The model under review builds one solid part; all positions refer to its coordinate system, in mm. A direction names the side the tool comes from. Round coordinates to 2 decimals unless told otherwise and drop trailing zeros. Order: outer loops, then holes, each group sorted by start corner. A loop starts at its lowest first (then second) coordinate and runs counter-clockwise, first axis right, second up. Notation, with made-up numbers: (-27.5, 76.25) -> (19.5, 76.25) arc R24 cw to (19.5, 96.25) -> close; hole circle Ø11 at (-39, -25). An arc over 180 degrees is marked (long way). Put each result on its own line as item: value. Start each with the question number.
from build123d import *

# Parameters (mm, degrees)
SKETCH2_R           = 37.5
SKETCH2_R_2         = 7.5
BOSS_EXTRUDE1_DEPTH = 7.5
SKETCH3_R           = 45
SKETCH3_R_2         = 37.5
BOSS_EXTRUDE2_DEPTH = 15
SKETCH4_R           = 42
SKETCH4_R_2         = 37.5
BOSS_EXTRUDE3_DEPTH = 10
SKETCH5_R           = 45
SKETCH5_R_2         = 42
SKETCH5_R_3         = 37.5
BOSS_EXTRUDE4_DEPTH = 20
SKETCH6_R           = 42
SKETCH6_R_2         = 37.5
BOSS_EXTRUDE5_DEPTH = 10
SKETCH7_R           = 45
SKETCH7_R_2         = 37.5
BOSS_EXTRUDE6_DEPTH = 15
FILLET1_R           = 5


with BuildPart() as part:
    # Sketch2 → Boss-Extrude1 (new body)
    with BuildSketch(Plane(origin=(0, 0, 0), x_dir=(1, 0, 0), z_dir=(0, 1, 0))):
        with BuildLine():
            ThreePointArc((8.95472604, 59.328010935), (-30, 51.961524227), (-55.856927646, 21.908985233))
            ThreePointArc((-55.856927646, 21.908985233), (-62.363007589, 17.536247736), (-70.05, 16))
            ThreePointArc((-70.05, 16), (-86.05, 0), (-70.05, -16))
            ThreePointArc((-70.05, -16), (-62.363007589, -17.536247736), (-55.856927646, -21.908985233))
            ThreePointArc((-55.856927646, -21.908985233), (-30, -51.961524227), (8.95472604, -59.328010935))
            ThreePointArc((8.95472604, -59.328010935), (15.994667768, -62.776072696), (21.168593539, -68.665079535))
            ThreePointArc((21.168593539, -68.665079535), (43.025, -74.521485996), (48.881406461, -52.665079535))
            ThreePointArc((48.881406461, -52.665079535), (46.368339821, -45.23982496), (46.902201606, -37.419025702))
            ThreePointArc((46.902201606, -37.419025702), (60, 0), (46.902201606, 37.419025702))
            ThreePointArc((46.902201606, 37.419025702), (46.368339821, 45.23982496), (48.881406461, 52.665079535))
            ThreePointArc((48.881406461, 52.665079535), (43.025, 74.521485996), (21.168593539, 68.665079535))
            ThreePointArc((21.168593539, 68.665079535), (15.994667768, 62.776072696), (8.95472604, 59.328010935))
        make_face()
        with Locations(Location((0, 0, 0), (0, 0, 270))):
            Circle(SKETCH2_R, mode=Mode.SUBTRACT)
        with Locations(Location((-70.05, 0, 0), (0, 0, 270))):
            Circle(SKETCH2_R_2, mode=Mode.SUBTRACT)
        with Locations(Location((35.025, 60.665079535, 0), (0, 0, 270))):
            Circle(SKETCH2_R_2, mode=Mode.SUBTRACT)
        with Locations(Location((35.025, -60.665079535, 0), (0, 0, 270))):
            Circle(SKETCH2_R_2, mode=Mode.SUBTRACT)
    extrude(amount=BOSS_EXTRUDE1_DEPTH)

    # Sketch3 → Boss-Extrude2 (add)
    with BuildSketch(Plane(origin=(0, 7.5, 0), x_dir=(1, 0, 0), z_dir=(0, 1, 0))):
        with Locations(Location((0, 0, 0), (0, 0, 90))):
            Circle(SKETCH3_R)
        with Locations(Location((0, 0, 0), (0, 0, 270))):
            Circle(SKETCH3_R_2, mode=Mode.SUBTRACT)
    extrude(amount=BOSS_EXTRUDE2_DEPTH)

    # Sketch4 → Boss-Extrude3 (add)
    with BuildSketch(Plane(origin=(0, 22.5, 0), x_dir=(1, 0, 0), z_dir=(0, 1, 0))):
        with Locations(Location((0, 0, 0), (0, 0, 270))):
            Circle(SKETCH4_R)
        with Locations(Location((0, 0, 0), (0, 0, 270))):
            Circle(SKETCH4_R_2, mode=Mode.SUBTRACT)
    extrude(amount=BOSS_EXTRUDE3_DEPTH)

    # Sketch5 → Boss-Extrude4 (add)
    # profile 1 of 2: a face of its own
    with BuildSketch(Plane(origin=(0, 32.5, 0), x_dir=(1, 0, 0), z_dir=(0, 1, 0))):
        with Locations(Location((0, 0, 0), (0, 0, 90))):
            Circle(SKETCH5_R)
        with Locations(Location((0, 0, 0), (0, 0, 270))):
            Circle(SKETCH5_R_2, mode=Mode.SUBTRACT)
    # profile 2 of 2: a face of its own
    with BuildSketch(Plane(origin=(0, 32.5, 0), x_dir=(1, 0, 0), z_dir=(0, 1, 0))):
        with Locations(Location((0, 0, 0), (0, 0, 270))):
            Circle(SKETCH5_R_2)
        with Locations(Location((0, 0, 0), (0, 0, 270))):
            Circle(SKETCH5_R_3, mode=Mode.SUBTRACT)
    extrude(amount=BOSS_EXTRUDE4_DEPTH)

    # Sketch6 → Boss-Extrude5 (add)
    with BuildSketch(Plane(origin=(0, 52.5, 0), x_dir=(1, 0, 0), z_dir=(0, 1, 0))):
        with Locations(Location((0, 0, 0), (0, 0, 270))):
            Circle(SKETCH6_R)
        with Locations(Location((0, 0, 0), (0, 0, 270))):
            Circle(SKETCH6_R_2, mode=Mode.SUBTRACT)
    extrude(amount=BOSS_EXTRUDE5_DEPTH)

    # Sketch7 → Boss-Extrude6 (add)
    with BuildSketch(Plane(origin=(0, 62.5, 0), x_dir=(1, 0, 0), z_dir=(0, 1, 0))):
        with Locations(Location((0, 0, 0), (0, 0, 90))):
            Circle(SKETCH7_R)
        with Locations(Location((0, 0, 0), (0, 0, 270))):
            Circle(SKETCH7_R_2, mode=Mode.SUBTRACT)
    extrude(amount=BOSS_EXTRUDE6_DEPTH)

    # Fillet1
    fillet1_edges = [part.edges().sort_by_distance(p)[0] for p in [
        (0, 7.5, 45),
    ]]
    fillet(fillet1_edges, radius=FILLET1_R)


solid = part.part
Q1. Take a section at D-D on x = -75.5. Give the boundary of the cut face in (y, z), and give its area (3 significant figures).
Q2. Draft analysis for pull direction X (two halves, no side actions). For faces 1 (the face through (40, 22.5, 14)), 2 (the face through (32.15, 3.7, -53.74)), 3 (the face through (43.33, 3.7, -74.34)), 4 (the face through (46.354, 3.698, -45.13)), state which applies: +X half, -X half, draft (parallel to the pull), parting line (faces both ways), or undercut.
Q3. Take a section at B-B on z = 0. State how many separate pieces and enclosed holes the cut face has, and give its area (3 significant figures).
Q4. For faces 5 (the face through (17.235, 69.895, -41.569)), 6 (the face through (-35, 0, -17)), 7 (the face through (40, 62.5, 14)), list the 3-axis set-ups (+Z, -Z, +X, -X, +Y, -Y) from which the entire face can be reached by the end or side of a thin tool; tool diameter is ignored.
Q5. Clearance check with flat-ended pins moving along their axes: pin 1 Ø1.5 at (x, y) = (-38.5, 57.5) entering from +Z; pin 2 Ø13.5 at (x, z) = (-70.05, 0) entering from -Y; pin 3 Ø8 at (x, y) = (-4.5, 8) entering from +Z; pin 4 Ø12 at (x, y) = (11.5, 24) entering from -Z. State where each tip first meets the part, or that it passes through.
Q6. Wall thickness on probe 1 along X at (y, z) = (66, -0.5); probe 2 along X at (y, z) = (4, 0); probe 3 along X at (y, z) = (43.5, -24.5): over which ranges is each line inside the solid? List them lowest first. Write a range as [from, to].
Q7. Take a section at C-C on y = 28.5. Give the boundary of the cut face in (x, z), and give its area (3 significant figures).
Calculated:
1. outline: (0, -15.04) -> (7.5, -15.04) -> (7.5, -5.15) -> (0, -5.15) -> close; (0, 5.15) -> (7.5, 5.15) -> (7.5, 15.04) -> (0, 15.04) -> close
1. area: 148 mm²
2. face 1: draft
2. face 2: undercut
2. face 3: parting line
2. face 4: +X half
3. separate pieces: 3
3. enclosed holes: 0
3. area: 1,360 mm²
4. face 5: +Y
4. face 6: +Z, -Z, +X, -X, -Y
4. face 7: none
5. pin 1: stops at z = 18.41
5. pin 2: passes through
5. pin 3: stops at z = 60
5. pin 4: stops at z = -44.64
6. probe 1: x = [-45, -37.5], [37.5, 45]
6. probe 2: x = [-86.05, -77.55], [-62.55, -37.5], [37.5, 60]
6. probe 3: x = [-37.75, -28.39], [28.39, 37.75]
7. outline: circle Ø84 at (0, 0); hole circle Ø75 at (0, 0)
7. area: 1,120 mm²
